Geometry check sheet. Reference: the model listing, model coordinates, mm. Give positions to 0.01 mm unless a question says otherwise; leave off trailing zeros. Loops run counter-clockwise (first coordinate to the right, second up) from the corner with the lowest first, then second, coordinate; pieces in that order, holes last. Notation, with made-up numbers: (1.25, 9) -> (27.25, 9) arc R12 cw to (27.25, 27) -> close; hole circle Ø2 at (85.25, -9.5). An arc over 180 degrees is marked (long way). Write item = value, one per line.
```python
from build123d import *

# Parameters (mm, degrees)
F0_R     = 6.35
F1_DEPTH = 6.35


with BuildPart() as f1:
    # F0 (on Top) → F1 (new body)
    with BuildSketch(Plane.XY):
        with BuildLine():
            ThreePointArc((6.300195, 24.60625), (0, 19.05), (-6.300195, 24.60625))
            ThreePointArc((-6.300195, 24.60625), (-17.960512, 17.960512), (-24.60625, 6.300195))
            ThreePointArc((-24.60625, 6.300195), (-19.05, 0), (-24.60625, -6.300195))
            ThreePointArc((-24.60625, -6.300195), (-17.960512, -17.960512), (-6.300195, -24.60625))
            ThreePointArc((-6.300195, -24.60625), (0, -19.05), (6.300195, -24.60625))
            ThreePointArc((6.300195, -24.60625), (17.960512, -17.960512), (24.60625, -6.300195))
            ThreePointArc((24.60625, -6.300195), (19.05, 0), (24.60625, 6.300195))
            ThreePointArc((24.60625, 6.300195), (17.960512, 17.960512), (6.300195, 24.60625))
        make_face()
        with Locations((-11.22532, -11.22532)):
            Circle(F0_R, mode=Mode.SUBTRACT)
        with Locations((11.22532, -11.22532)):
            Circle(F0_R, mode=Mode.SUBTRACT)
        with Locations((-11.22532, 11.22532)):
            Circle(F0_R, mode=Mode.SUBTRACT)
        Circle(F0_R, mode=Mode.SUBTRACT)
        with Locations((11.22532, 11.22532)):
            Circle(F0_R, mode=Mode.SUBTRACT)
    extrude(amount=F1_DEPTH)


solid = f1.part
```
Item 1: Gauge pin test, flat ends, axial feed: pin 1 (3 mm diameter, centred on x = -14, z = 3, fed in from -Y); pin 2 (1.5 mm diameter, centred on y = -15.5, z = 5, fed in from -X); pin 3 (3 mm diameter, centred on x = 14, z = 0.5, fed in from +Y). Record the tip position at first contact, or that the pin passes through.
Answer:
pin_1 = -22.11
pin_2 = -20.68
pin_3 = 22.11
Item 2: Draft check along Y on faces 1 (the cylindrical face through (-5.36, -13.66, 3.13)), 2 (the cylindrical face through (-1.38, -6.2, 3.13)), 3 (the cylindrical face through (0.13, 19.05, 3.13)), 4 (the cylindrical face through (17.83, -18.09, 3.13)). Enter one of: +Y half, -Y half, draft (parallel to the pull), parting line (faces both ways), or undercut.
Answer:
face_1 = undercut
face_2 = undercut
face_3 = +Y half
face_4 = -Y half
Item 3: Section check A-A, the plane x = 0. Record the cut outline in (y, z).
Answer:
outline = (-19.05, 0) -> (-6.35, 0) -> (-6.35, 6.35) -> (-19.05, 6.35) -> close; (6.35, 0) -> (19.05, 0) -> (19.05, 6.35) -> (6.35, 6.35) -> close
Item 4: Section check D-D, the plane x = -11. Record the cut outline in (y, z), plus the area to 3 significant figures.
Answer:
outline = (-22.89, 0) -> (-17.57, 0) -> (-17.57, 6.35) -> (-22.89, 6.35) -> close; (-4.88, 0) -> (4.88, 0) -> (4.88, 6.35) -> (-4.88, 6.35) -> close; (17.57, 0) -> (22.89, 0) -> (22.89, 6.35) -> (17.57, 6.35) -> close
area = 130 mm^2
Item 5: Thickness scan on L1, parallel to X at y = 8, z = 2.5; L2, parallel to X at y = -8.5, z = 6; L3, parallel to Y at x = -10, z = 3.75. Record the ranges inside material, lowest first. Write a range as [from, to].
Answer:
L1 = [-24.11, -16.7], [-5.76, 5.76], [16.7, 24.11]
L2 = [-23.94, -16.96], [-5.49, 5.49], [16.96, 23.94]
L3 = [-23.35, -17.46], [-4.99, 4.99], [17.46, 23.35]
Item 6: Section check C-C, the plane z = 2.5. Record the cut outline in (x, y), plus the area to 3 significant figures.
Answer:
outline = (-24.61, -6.3) arc R25.4 ccw to (-6.3, -24.61) arc R6.35 cw to (6.3, -24.61) arc R25.4 ccw to (24.61, -6.3) arc R6.35 cw to (24.61, 6.3) arc R25.4 ccw to (6.3, 24.61) arc R6.35 cw to (-6.3, 24.61) arc R25.4 ccw to (-24.61, 6.3) arc R6.35 cw to start; hole circle Ø12.7 at (-11.23, -11.23); hole circle Ø12.7 at (-11.23, 11.23); hole circle Ø12.7 at (0, 0); hole circle Ø12.7 at (11.23, -11.23); hole circle Ø12.7 at (11.23, 11.23)
area = 1,150 mm^2
